Can you work these out from the model? Positions are in its coordinate system, mm. Face numbers are marked on the shaded views. A direction names the side the tool comes from. Give positions to 0.01 mm unless a question says otherwise; leave off trailing zeros. Order: outer loops, then holes, each group sorted by start corner. A loop starts at its lowest first (then second) coordinate and runs counter-clockwise, first axis right, second up. Notation, with made-up numbers: (-26.75, 84) - (6.25, 84) arc R5 ccw to (6.25, 89) - close; hole circle Ø9 at (62.25, -37). An arc over 180 degrees is marked (long way). Return JSON: item names as keys, results as strings.
```python
from build123d import *

# Parameters (mm, degrees)
SKETCH1_W           = 200
SKETCH1_H           = 200
SKETCH1_W_2         = 20
SKETCH1_H_2         = 80
BOSS_EXTRUDE1_DEPTH = 50
SHELL1_START        = 20.678946788
SHELL1_OUTLINE_W    = 30
SHELL1_OUTLINE_H    = 160
SHELL1_DEPTH        = 100
SHELL1_START_2      = -39.321053212
SHELL1_2_OUTLINE_W  = 30
SHELL1_2_OUTLINE_H  = 20
SHELL1_2_DEPTH      = 60
SKETCH4_W           = 60
SKETCH4_H           = 120
CUT_EXTRUDE1_DEPTH  = 30
BOSS_EXTRUDE2_DEPTH = 50
SKETCH6_W           = 20
SKETCH6_H           = 45
CUT_EXTRUDE2_DEPTH  = 30
SKETCH7_R           = 10
CUT_EXTRUDE3_DEPTH  = 28
SKETCH8_W           = 160.292931591
SKETCH8_H           = 30
CUT_EXTRUDE4_DEPTH  = 213


# Read off the part's stored shape, not the designer's step: Shell1
with BuildPart() as part:
    # Sketch1 → Boss-Extrude1 (new body)
    with BuildSketch(Plane(origin=(0, 0, 0), x_dir=(1, 0, 0), z_dir=(0, 1, 0))):
        with Locations((40.678946788, 74.932071062)):
            Rectangle(SKETCH1_W, SKETCH1_H)
        with Locations((-9.321053212, 74.932071062)):
            Rectangle(SKETCH1_W_2, SKETCH1_H_2, mode=Mode.SUBTRACT)
    extrude(amount=BOSS_EXTRUDE1_DEPTH)

    # Shell1 outline → Shell1 (cut)
    with BuildSketch(Plane.YZ.offset(SHELL1_START)):
        with Locations((35, -74.932071062)):
            Rectangle(SHELL1_OUTLINE_W, SHELL1_OUTLINE_H)
    extrude(amount=SHELL1_DEPTH, mode=Mode.SUBTRACT)

    # Shell1 2 outline → Shell1 2 (cut)
    with BuildSketch(Plane.YZ.offset(SHELL1_START_2)):
        with Locations((35, -144.932071062)):
            Rectangle(SHELL1_2_OUTLINE_W, SHELL1_2_OUTLINE_H)
        with Locations((35, -4.932071062)):
            Rectangle(SHELL1_2_OUTLINE_W, SHELL1_2_OUTLINE_H)
    extrude(amount=SHELL1_2_DEPTH, mode=Mode.SUBTRACT)

    # Sketch4 → Cut-Extrude1 (cut)
    with BuildSketch(Plane(origin=(0, 50, 0), x_dir=(1, 0, 0), z_dir=(0, 1, 0))):
        with Locations((-9.321053212, 74.932071062)):
            Rectangle(SKETCH4_W, SKETCH4_H)
    extrude(amount=-CUT_EXTRUDE1_DEPTH, mode=Mode.SUBTRACT)

    # Sketch5 → Boss-Extrude2 (add)
    with BuildSketch(Plane.XZ):
        Polygon((40.678946788, 25.067928938), (15.678946788, 25.067928938), (0.678946788, 50.067928938), (80.678946788, 50.067928938), (65.678946788, 25.067928938), align=None)
    boss_extrude2 = extrude(amount=-BOSS_EXTRUDE2_DEPTH)

    # Sketch6 → Cut-Extrude2 (cut)
    with BuildSketch(Plane(origin=(0, 50, 0), x_dir=(1, 0, 0), z_dir=(0, 1, 0))):
        with Locations((40.678946788, -27.567928938)):
            Rectangle(SKETCH6_W, SKETCH6_H)
    cut_extrude2 = extrude(amount=-CUT_EXTRUDE2_DEPTH, mode=Mode.SUBTRACT)

    # Mirror1: Boss-Extrude2, Cut-Extrude2 across plane
    add(boss_extrude2.mirror(Plane.XY.offset(-74.932071062)))
    add(cut_extrude2.mirror(Plane.XY.offset(-74.932071062)), mode=Mode.SUBTRACT)

    # Sketch7 → Cut-Extrude3 (cut)
    with BuildSketch(Plane(origin=(0, 0, 0), x_dir=(-1, 0, 0), z_dir=(0, -1, 0))):
        with Locations(Location((-74.835730419, 71.684680876, 0), (0, 0, 90))):
            Circle(SKETCH7_R)
    extrude(amount=-CUT_EXTRUDE3_DEPTH, mode=Mode.SUBTRACT)

    # Sketch8 → Cut-Extrude4 (cut)
    with BuildSketch(Plane(origin=(140.678946788, 0, 0), x_dir=(0, 0, -1), z_dir=(1, 0, 0))):
        with Locations((74.785605266, 35)):
            Rectangle(SKETCH8_W, SKETCH8_H)
    extrude(amount=-CUT_EXTRUDE4_DEPTH, mode=Mode.SUBTRACT)


solid = part.part
```
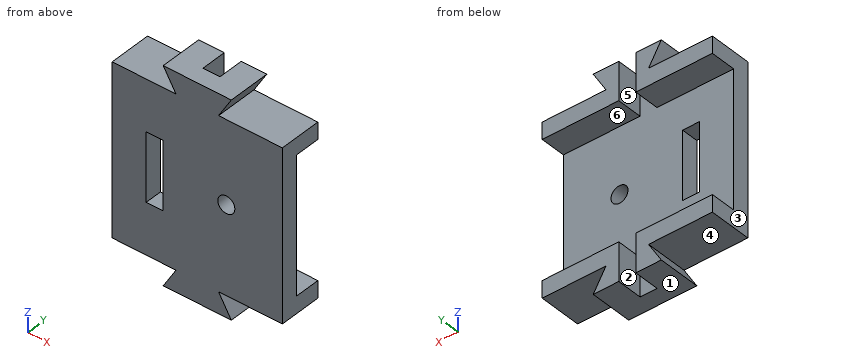
1. Suppose I cut it at A-A (x = -4.5). List the corners of the cut face in (y, z) for me.
Checks:
{"outline": "(0, -174.93) - (50, -174.93) - (50, -154.93) - (20, -154.93) - (20, -114.93) - (0, -114.93) - close; (0, -34.93) - (20, -34.93) - (20, 5.36) - (50, 5.36) - (50, 25.07) - (0, 25.07) - close"}
2. If I drill on L1, parallel to Z at x = 89.5, y = 46.5; L2, parallel to X at y = 37.5, z = 24; L3, parallel to X at y = 16, z = -110.5, over which ranges is the centre line in solid material (lowest first)? Write a range as [from, to].
Checks:
{"L1": "[-174.93, -154.93], [5.36, 25.07]", "L2": "[-59.32, 30.68], [50.68, 140.68]", "L3": "[-59.32, -19.32], [0.68, 140.68]"}
3. On a 3-axis mill with a long thin cutter (end or side, diameter ignored), from which of +Z, -Z, +X, -X, +Y, -Y can I reach the whole of each face in a straight line? I mean the marked faces 4, 5 and 6. Say none if no direction works.
Checks:
{"face 4": "-X, +Y, -Y", "face 5": "+Z, -Z, +Y", "face 6": "+X, -X, +Y"}
4. Suppose I cut it at D-D (x = 26). List the corners of the cut face in (y, z) for me, plus the area to 3 significant figures.
Checks:
{"outline": "(0, -199.93) - (50, -199.93) - (50, -154.93) - (20, -154.93) - (20, 5.36) - (50, 5.36) - (50, 50.07) - (0, 50.07) - close", "area": "7,690 mm^2"}
5. Suppose I cut it at C-C (z = -96.5). List the corners of the cut face in (x, y) for me, plus the area to 3 significant figures.
Checks:
{"outline": "(-59.32, 0) - (-19.32, 0) - (-19.32, 20) - (-59.32, 20) - close; (0.68, 0) - (140.68, 0) - (140.68, 20) - (0.68, 20) - close", "area": "3,600 mm^2"}
6. For pin 1 Ø10 at (x, z) = (50.5, -45.5) entering from +Y; pin 2 Ø12 at (x, z) = (74.84, -71.68) entering from +Y; pin 3 Ø6 at (x, y) = (-11.5, 14.5) entering from +Z; pin 4 Ø15 at (x, y) = (-30.5, 22.5) entering from -Z, each with a flat end and sliding along its axis, tell me the tip position at first contact or that it passes through.
Checks:
{"pin 1": "y = 20", "pin 2": "through", "pin 3": "z = 25.07", "pin 4": "z = -174.93"}
7. Thinking about a two-plate mould opening in X: for the marked faces 1, 2 and 3, which applies, +X half, -X half, draft (parallel to the pull), parting line (faces both ways), or undercut?
Checks:
{"face 1": "draft", "face 2": "undercut", "face 3": "-X half"}
8. Suppose I cut it at B-B (y = 23). List the corners of the cut face in (x, z) for me, plus the area to 3 significant figures.
Checks:
{"outline": "(-59.32, -174.93) - (15.68, -174.93) - (0.68, -199.93) - (30.68, -199.93) - (30.68, -154.93) - (-59.32, -154.93) - close; (-59.32, 5.36) - (30.68, 5.36) - (30.68, 50.07) - (0.68, 50.07) - (15.68, 25.07) - (-59.32, 25.07) - close; (50.68, -199.93) - (80.68, -199.93) - (65.68, -174.93) - (140.68, -174.93) - (140.68, -154.93) - (50.68, -154.93) - close; (50.68, 5.36) - (140.68, 5.36) - (140.68, 25.07) - (65.68, 25.07) - (80.68, 50.07) - (50.68, 50.07) - close", "area": "9,400 mm^2"}
